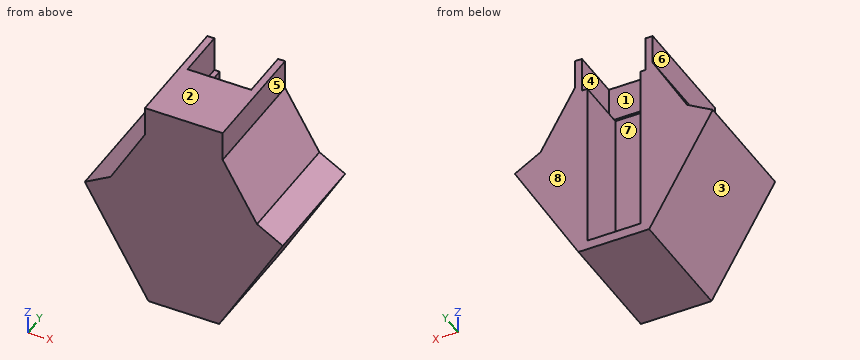
Autodesk Inventor part; units mm, degrees
ref_plane "YZ Plane" through (0, 0, 0) normal (1, 0, 0) x (0, 1, 0)
ref_plane "XZ Plane" through (0, 0, 0) normal (0, 1, 0) x (-1, 0, 0)
ref_plane "XY Plane" through (0, 0, 0) normal (0, 0, 1) x (1, 0, 0)
sketch "スケッチ1" plane through (0, 0, 0) normal (0, 1, 0) x (-1, 0, 0)
  line L0 (135, 77.9423) -> (-135, 77.9423)
  line L1 (-135, 77.9423) -> (0, -155.8846)
  line L2 (0, -155.8846) -> (135, 77.9423)
  line L3 (135, 77.9423) -> (-67.5, -38.9711)
  line L4 (75, 77.9423) -> (105, 25.9808)
  line L5 (30, -103.923) -> (-30, -103.923)
  line L6 (-105, 25.9808) -> (-75, 77.9423)
  line L7 (0, 77.9423) -> (0, -155.8846)
  line L8 (-135, 77.9423) -> (67.5, -38.9711)
  line L9 (-33, 77.9423) -> (-33, 52.6884)
  line L10 (-33, 52.6884) -> (-62.1295, 2.2346)
  line L11 (-62.1295, 2.2346) -> (-84, -10.3923)
  line L12 (27, 77.9423) -> (-27, 77.9423)
  line L13 (-27, 77.9423) -> (-27, 47.9423)
  line L14 (-27, 47.9423) -> (27, 47.9423)
  line L15 (27, 47.9423) -> (27, 77.9423)
  point P0 (0, 0)
  point P1 (0, 77.9423)
  point P2 (0, 47.9423)
  dimension "d0" = 270
  dimension "d2" = 30
  dimension "d5" = 42
  dimension "d6" = 49
  dimension "d9" = 54
  dimension "d14" = 30
extrude "押し出し1" add sketch "スケッチ1" along normal blind 100 contours L4 L3 L7 L14 L15 L0 | L2 L8 L3 L4 | L15 L14 L7 L0 | L2 L5 L7 L8 | L7 L5 L1 L3 | L8 L10 L9 L0 L13 L14 L7 | L3 L1 L11 L10 L8 | L7 L14 L13 L0 | L10 L11 L1 L6 L8 | L8 L6 L0 L9 L10
extrude "押し出し2" cut sketch "スケッチ1" along normal blind 100 contours L10 L11 L1 L6 L8 | L8 L6 L0 L9 L10
mirror "ミラー1" about plane through (0, 0, 0) normal (1, 0, 0) of "押し出し2"
extrude "押し出し3" cut sketch "スケッチ1" along normal blind 100 contours L15 L14 L7 L0 | L7 L14 L13 L0
extrude "押し出し4" add sketch "スケッチ1" along normal blind 57 contours L15 L14 L7 L0 | L7 L14 L13 L0
sketch "スケッチ2" plane through (0, 100, 0) normal (0, 1, 0) x (1, 0, 0)
  line L0 (-27, -47.9423) -> (27, -47.9423)
  line L1 (-22.5, -47.9423) -> (22.5, -47.9423)
  line L2 (22.5, -47.9423) -> (22.5, 95.923)
  line L3 (22.5, 95.923) -> (-22.5, 95.923)
  line L4 (-22.5, 95.923) -> (-22.5, -47.9423)
  line L5 (30, 103.923) -> (-30, 103.923)
  point P0 (0, 0)
  point P1 (0, -47.9423)
  dimension "d15" = 45
  dimension "d16" = 8
extrude "押し出し5" cut sketch "スケッチ2" against normal blind 45
properties part number "cover"
Check sheet for the modelled part. Datum: model origin and axes. Units: mm. Face numbers are marked on the shaded views. A direction names the side the tool comes from. Round coordinates to 2 decimals unless told otherwise and drop trailing zeros. Loops run counter-clockwise (first coordinate to the right, second up) from the corner with the lowest first, then second, coordinate; pieces in that order, holes last. Notation, with made-up numbers: (-2, -35) -> (34, -35) arc R26 cw to (34, -6) -> close; hole circle Ø3 at (76, 86.25). An arc over 180 degrees is marked (long way). Answer in a Markdown table with one row per item.
Q1. Sectioned sample at D-D on x = -56.5. Enter the section's corners in (y, z), then the cut area to 3 significant figures.
Data:
| item | result |
|---|---|
| outline | (0, -58.02) -> (100, -58.02) -> (100, 11.99) -> (0, 11.99) -> close |
| area | 7,000 mm^2 |
Q2. Go/stop test with flat-tipped pins: P1, Ø24, axis at y = 81, z = 60.5, coming from the +X side; P2, Ø3, axis at y = 49.5, z = 30.5, coming from the -X side; P3, Ø1, axis at y = 61.5, z = 44.5, coming from the -X side; P4, Ø12, axis at x = 44, z = 49, coming from the -Y side. Record where each tip stops, or that it passes through.
Data:
| item | result |
|---|---|
| P1 | stops at x = 35.42 |
| P2 | stops at x = -46.68 |
| P3 | stops at x = -38.02 |
| P4 | passes through |
Q3. Release check for a two-part mould opening along X. For the marked faces 1, 2 and 3 record: released by +X, released by -X, zero draft, split by the parting line, or undercut.
Data:
| item | result |
|---|---|
| face 1 | undercut |
| face 2 | zero draft |
| face 3 | released by -X |
Q4. Sectioned sample at A-A on x = -19. Enter the section's corners in (y, z), then the cut area to 3 significant figures.
Data:
| item | result |
|---|---|
| outline | (0, -103.92) -> (100, -103.92) -> (100, -95.92) -> (55, -95.92) -> (55, 47.94) -> (57, 47.94) -> (57, 77.94) -> (0, 77.94) -> close |
| area | 10,400 mm^2 |
Q5. Thickness scan on L1, parallel to X at y = 78, z = 55.5; L2, parallel to Y at x = 20.5, z = -93.5; L3, parallel to Z at x = 15.5, y = 78.5. Record the ranges inside material, lowest first.
Data:
| item | result |
|---|---|
| L1 | x = -33 to -27, 27 to 33 |
| L2 | y = 0 to 55 |
| L3 | z = -103.92 to -95.92 |
Q6. Sectioned sample at C-C on y = 67.5. Enter the section's corners in (x, z).
Data:
| item | result |
|---|---|
| outline | (-84, -10.39) -> (-30, -103.92) -> (30, -103.92) -> (84, -10.39) -> (62.13, 2.23) -> (33, 52.69) -> (33, 77.94) -> (27, 77.94) -> (27, 47.94) -> (22.5, 47.94) -> (22.5, -95.92) -> (-22.5, -95.92) -> (-22.5, 47.94) -> (-27, 47.94) -> (-27, 77.94) -> (-33, 77.94) -> (-33, 52.69) -> (-62.13, 2.23) -> close |
Q7. Sectioned sample at B-B on z = 5. Enter the section's corners in (x, y), then the cut area to 3 significant figures.
Data:
| item | result |
|---|---|
| outline | (-60.53, 0) -> (60.53, 0) -> (60.53, 100) -> (22.5, 100) -> (22.5, 55) -> (-22.5, 55) -> (-22.5, 100) -> (-60.53, 100) -> close |
| area | 10,100 mm^2 |
Q8. Set-up check for the marked faces 4, 5, 6, 7 and 8: record each of +Z, -Z, +X, -X, +Y, -Y from which the full face is reachable in a straight line by a thin tool's end or side.
Data:
| item | result |
|---|---|
| face 4 | +Z, +Y |
| face 5 | +Z, +X, +Y, -Y |
| face 6 | +Z, -X, +Y, -Y |
| face 7 | +Y |
| face 8 | +Z, -Z, +X, -X, +Y |
